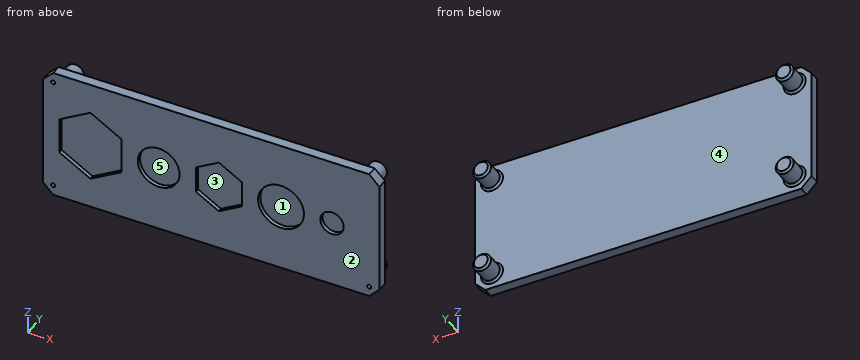
```python
from build123d import *

# Parameters (mm, degrees)
SKETCH2_W           = 165
SKETCH2_H           = 65
BOSS_EXTRUDE1_DEPTH = 5
SKETCH3_R           = 4.4
BOSS_EXTRUDE2_DEPTH = 10
CHAMFER1_SIZE       = 1
CHAMFER2_SIZE       = 5
SKETCH4_R           = 1
CUT_EXTRUDE1_DEPTH  = 2
SKETCH5_R           = 10.25
SKETCH5_R_2         = 11.25
SKETCH5_R_3         = 5.75
CUT_EXTRUDE2_DEPTH  = 2


with BuildPart() as part:
    # Sketch2 → Boss-Extrude1 (new body)
    with BuildSketch(Plane(origin=(0, 0, 0), x_dir=(1, 0, 0), z_dir=(0, 1, 0))):
        Rectangle(SKETCH2_W, SKETCH2_H)
    extrude(amount=BOSS_EXTRUDE1_DEPTH)

    # Sketch3 → Boss-Extrude2 (add)
    with BuildSketch(Plane(origin=(0, 5, 0), x_dir=(1, 0, 0), z_dir=(0, 1, 0))):
        with Locations(Location((-74.245, 24.75, 0), (0, 0, 90))):
            Circle(SKETCH3_R)
        with Locations(Location((-74.245, -24.75, 0), (0, 0, 90))):
            Circle(SKETCH3_R)
        with Locations(Location((74.245, -24.75, 0), (0, 0, 90))):
            Circle(SKETCH3_R)
        with Locations(Location((74.245, 24.75, 0), (0, 0, 90))):
            Circle(SKETCH3_R)
    extrude(amount=BOSS_EXTRUDE2_DEPTH)

    # Chamfer1
    chamfer1_edges = [part.edges().sort_by_distance(p)[0] for p in [
        (-74.245, 5, -20.35),
        (-74.245, 15, -20.35),
        (-74.245, 5, 29.15),
        (-74.245, 15, 29.15),
        (74.245, 5, 29.15),
        (74.245, 15, 29.15),
        (74.245, 5, -20.35),
        (74.245, 15, -20.35),
    ]]
    chamfer(chamfer1_edges, length=CHAMFER1_SIZE)

    # Chamfer2
    chamfer2_edges = [part.edges().sort_by_distance(p)[0] for p in [
        (82.5, 2.5, 32.5),
        (-82.5, 2.5, 32.5),
        (-82.5, 2.5, -32.5),
        (82.5, 2.5, -32.5),
    ]]
    chamfer(chamfer2_edges, length=CHAMFER2_SIZE)

    # Sketch4 → Cut-Extrude1 (cut)
    with BuildSketch(Plane.XZ):
        with Locations(Location((-77.5, 27.5, 0), (0, 0, 270))):
            Circle(SKETCH4_R)
        with Locations(Location((-77.5, -27.5, 0), (0, 0, 270))):
            Circle(SKETCH4_R)
        with Locations(Location((77.5, -27.5, 0), (0, 0, 270))):
            Circle(SKETCH4_R)
    extrude(amount=-CUT_EXTRUDE1_DEPTH, mode=Mode.SUBTRACT)

    # Sketch5 → Cut-Extrude2 (cut)
    with BuildSketch(Plane.XZ):
        with Locations(Location((-25.75, 0, 0), (0, 0, 270))):
            Circle(SKETCH5_R)
        with Locations(Location((34.25, 0, 0), (0, 0, 270))):
            Circle(SKETCH5_R_2)
        with Locations(Location((59.25, 0, 0), (0, 0, 270))):
            Circle(SKETCH5_R_3)
        Polygon((-59.25, 17.60918321), (-74.5, 8.804591605), (-74.5, -8.804591605), (-59.25, -17.60918321), (-44, -8.804591605), (-44, 8.804591605), align=None)
        Polygon((15, -6.495190528), (15, 6.495190528), (3.75, 12.990381057), (-7.5, 6.495190528), (-7.5, -6.495190528), (3.75, -12.990381057), align=None)
    extrude(amount=-CUT_EXTRUDE2_DEPTH, mode=Mode.SUBTRACT)


solid = part.part
```
Can you work these out from the model? Positions are in its coordinate system, mm. Face numbers are marked on the shaded views. A direction names the side the tool comes from. Round coordinates to 2 decimals unless told otherwise and drop trailing zeros. Order: outer loops, then holes, each group sorted by start corner. A loop starts at its lowest first (then second) coordinate and runs counter-clockwise, first axis right, second up. Notation, with made-up numbers: (-29, 8.5) -> (4, 8.5) arc R15 cw to (4, 28.5) -> close; hole circle Ø5 at (61, -19.5). An arc over 180 degrees is marked (long way). Return JSON: item names as keys, results as strings. Group by question number.
1. If we section it at D-D, the plane x = -51.5: Write out the boundary of the cut face in (y, z), then the cut area to 3 significant figures.
2. If we section it at B-B, the plane x = -22: Write out the boundary of the cut face in (y, z).
3. If we section it at A-A, the plane z = -24.75: Write out the boundary of the cut face in (x, y) (3 decimals), then the cut area to 3 significant figures.
4. We'd pull the mould along Z, two halves only. Please class the marked faces 1, 2 and 3: released by +Z, released by -Z, zero draft, split by the parting line, or undercut.
5. Which directions (+Z, -Z, +X, -X, +Y, -Y) give clear straight access to the entire face, cutting with the end or side of a thin tool? Please do the marked faces 4 and 5.
6. I need wall thicknesses on line 1 (X direction, y = 1.5, z = 0); line 2 (Z direction, x = -77.5, y = 1.2); line 3 (X direction, y = 1.05, z = -27.5). Which ranges of each line are inside material? Lowest first, please. Write a range as [from, to].
7. If we section it at C-C, the plane z = 0: Write out the boundary of the cut face in (x, y).
8. Will these pins go through, and if not, where does the flat tip stop? pin 1 (2 mm diameter, centred on y = 12.5, z = 21.5, fed in from +X); pin 2 (18 mm diameter, centred on x = 34.25, z = 0, fed in from -Y); pin 3 (8 mm diameter, centred on y = 11.5, z = -21.5, fed in from +X) (3 decimals).
Output values:
{
 "1": {"outline": "(0, -32.5) -> (5, -32.5) -> (5, 32.5) -> (0, 32.5) -> (0, 13.13) -> (2, 13.13) -> (2, -13.13) -> (0, -13.13) -> close", "area": "272 mm²"},
 "2": {"outline": "(0, -32.5) -> (5, -32.5) -> (5, 32.5) -> (0, 32.5) -> (0, 9.54) -> (2, 9.54) -> (2, -9.54) -> (0, -9.54) -> close"},
 "3": {"outline": "(-82.5, 0) -> (82.5, 0) -> (82.5, 5) -> (79.645, 5) -> (78.645, 6) -> (78.645, 14) -> (77.645, 15) -> (70.845, 15) -> (69.845, 14) -> (69.845, 6) -> (68.845, 5) -> (-68.845, 5) -> (-69.845, 6) -> (-69.845, 14) -> (-70.845, 15) -> (-77.645, 15) -> (-78.645, 14) -> (-78.645, 6) -> (-79.645, 5) -> (-82.5, 5) -> close", "area": "1,000 mm²"},
 "4": {"face 1": "undercut", "face 2": "zero draft", "face 3": "undercut"},
 "5": {"face 4": "+Y", "face 5": "-Y"},
 "6": {"line 1": "[-82.5, -74.5], [-44, -36], [-15.5, -7.5], [15, 23], [45.5, 53.5], [65, 82.5]", "line 2": "[-32.5, -28.5], [-26.5, 26.5], [28.5, 32.5]", "line 3": "[-82.5, -78.5], [-76.5, 76.5], [78.5, 82.5]"},
 "7": {"outline": "(-82.5, 0) -> (-74.5, 0) -> (-74.5, 2) -> (-44, 2) -> (-44, 0) -> (-36, 0) -> (-36, 2) -> (-15.5, 2) -> (-15.5, 0) -> (-7.5, 0) -> (-7.5, 2) -> (15, 2) -> (15, 0) -> (23, 0) -> (23, 2) -> (45.5, 2) -> (45.5, 0) -> (53.5, 0) -> (53.5, 2) -> (65, 2) -> (65, 0) -> (82.5, 0) -> (82.5, 5) -> (-82.5, 5) -> close"},
 "8": {"pin 1": "x = 78.03", "pin 2": "y = 2", "pin 3": "x = 78.645"}
}
